Model file for the job. Use its own axes, mm. A direction names the side the tool comes from. Coordinates: 2 decimals unless noted, no trailing zeros. Loops run counter-clockwise (first coordinate to the right, second up) from the corner with the lowest first, then second, coordinate; pieces in that order, holes last. Notation, with made-up numbers: (76, 69.25) -> (87, 69.25) arc R10 cw to (87, 87.25) -> close; hole circle Ø5 at (5, -3.5). An arc over 180 degrees is marked (long way). Use one line per item in the form item = value.
```python
from build123d import *

# Parameters (mm, degrees)
MODEL_W             = 8.001
MODEL_H             = 8.001
BOSS_EXTRUDE2_DEPTH = 6.35


with BuildPart() as part:
    # Model → Boss-Extrude2 (new body)
    with BuildSketch(Plane.XY):
        Polygon((419.1, 87.376), (419.1, 71.374), (436.88, 71.374), (436.88, 63.5), (398.78, 0), (0, 0), (0, 95.25), (436.88, 95.25), (436.88, 87.376), align=None)
        with Locations((70.891200524, 88.9)):
            Rectangle(MODEL_W, MODEL_H, mode=Mode.SUBTRACT)
        Polygon((235.853706977, 81.865965064), (235.938184476, 73.865411048), (227.937630461, 73.780933549), (227.853152962, 81.781487564), align=None, mode=Mode.SUBTRACT)
        with BuildLine():
            Line((171.232102448, 6.35), (215.9, 6.35))
            ThreePointArc((215.9, 6.35), (220.390128061, 8.209871939), (222.25, 12.7))
            Line((222.25, 12.7), (222.25, 57.367897552))
            ThreePointArc((222.25, 57.367897552), (220.682015918, 59.714551565), (217.913948776, 59.163948776))
            Line((217.913948776, 59.163948776), (169.436051224, 10.686051224))
            ThreePointArc((169.436051224, 10.686051224), (168.885448435, 7.917984082), (171.232102448, 6.35))
        make_face(mode=Mode.SUBTRACT)
        with BuildLine():
            Line((234.95, 57.367897552), (234.95, 12.7))
            ThreePointArc((234.95, 12.7), (236.809871939, 8.209871939), (241.3, 6.35))
            Line((241.3, 6.35), (285.967897552, 6.35))
            ThreePointArc((285.967897552, 6.35), (288.314551565, 7.917984082), (287.763948776, 10.686051224))
            Line((287.763948776, 10.686051224), (239.286051224, 59.163948776))
            ThreePointArc((239.286051224, 59.163948776), (236.517984082, 59.714551565), (234.95, 57.367897552))
        make_face(mode=Mode.SUBTRACT)
        with BuildLine():
            Line((294.113948776, 17.036051224), (245.636051224, 65.513948776))
            ThreePointArc((245.636051224, 65.513948776), (245.085448435, 68.282015918), (247.432102448, 69.85))
            Line((247.432102448, 69.85), (292.1, 69.85))
            ThreePointArc((292.1, 69.85), (296.590128061, 67.990128061), (298.45, 63.5))
            Line((298.45, 63.5), (298.45, 18.832102448))
            ThreePointArc((298.45, 18.832102448), (296.882015918, 16.485448435), (294.113948776, 17.036051224))
        make_face(mode=Mode.SUBTRACT)
        with BuildLine():
            Line((323.632102448, 6.35), (368.3, 6.35))
            ThreePointArc((368.3, 6.35), (372.790128061, 8.209871939), (374.65, 12.7))
            Line((374.65, 12.7), (374.65, 57.367897552))
            ThreePointArc((374.65, 57.367897552), (373.082015918, 59.714551565), (370.313948776, 59.163948776))
            Line((370.313948776, 59.163948776), (321.836051224, 10.686051224))
            ThreePointArc((321.836051224, 10.686051224), (321.285448435, 7.917984082), (323.632102448, 6.35))
        make_face(mode=Mode.SUBTRACT)
        with BuildLine():
            Line((18.832102448, 6.35), (63.5, 6.35))
            ThreePointArc((63.5, 6.35), (67.990128061, 8.209871939), (69.85, 12.7))
            Line((69.85, 12.7), (69.85, 57.367897552))
            ThreePointArc((69.85, 57.367897552), (68.282015918, 59.714551565), (65.513948776, 59.163948776))
            Line((65.513948776, 59.163948776), (17.036051224, 10.686051224))
            ThreePointArc((17.036051224, 10.686051224), (16.485448435, 7.917984082), (18.832102448, 6.35))
        make_face(mode=Mode.SUBTRACT)
        with BuildLine():
            Line((82.55, 57.367897552), (82.55, 12.7))
            ThreePointArc((82.55, 12.7), (84.409871939, 8.209871939), (88.9, 6.35))
            Line((88.9, 6.35), (133.567897552, 6.35))
            ThreePointArc((133.567897552, 6.35), (135.914551565, 7.917984082), (135.363948776, 10.686051224))
            Line((135.363948776, 10.686051224), (86.886051224, 59.163948776))
            ThreePointArc((86.886051224, 59.163948776), (84.117984082, 59.714551565), (82.55, 57.367897552))
        make_face(mode=Mode.SUBTRACT)
        with BuildLine():
            Line((93.236051224, 65.513948776), (141.713948776, 17.036051224))
            ThreePointArc((141.713948776, 17.036051224), (144.482015918, 16.485448435), (146.05, 18.832102448))
            Line((146.05, 18.832102448), (146.05, 63.5))
            ThreePointArc((146.05, 63.5), (144.190128061, 67.990128061), (139.7, 69.85))
            Line((139.7, 69.85), (95.032102448, 69.85))
            ThreePointArc((95.032102448, 69.85), (92.685448435, 68.282015918), (93.236051224, 65.513948776))
        make_face(mode=Mode.SUBTRACT)
        with BuildLine():
            Line((163.086051224, 17.036051224), (211.563948776, 65.513948776))
            ThreePointArc((211.563948776, 65.513948776), (212.114551565, 68.282015918), (209.767897552, 69.85))
            Line((209.767897552, 69.85), (165.1, 69.85))
            ThreePointArc((165.1, 69.85), (160.609871939, 67.990128061), (158.75, 63.5))
            Line((158.75, 63.5), (158.75, 18.832102448))
            ThreePointArc((158.75, 18.832102448), (160.317984082, 16.485448435), (163.086051224, 17.036051224))
        make_face(mode=Mode.SUBTRACT)
        with BuildLine():
            Line((315.486051224, 17.036051224), (363.963948776, 65.513948776))
            ThreePointArc((363.963948776, 65.513948776), (364.514551565, 68.282015918), (362.167897552, 69.85))
            Line((362.167897552, 69.85), (317.5, 69.85))
            ThreePointArc((317.5, 69.85), (313.009871939, 67.990128061), (311.15, 63.5))
            Line((311.15, 63.5), (311.15, 18.832102448))
            ThreePointArc((311.15, 18.832102448), (312.717984082, 16.485448435), (315.486051224, 17.036051224))
        make_face(mode=Mode.SUBTRACT)
        with BuildLine():
            Line((6.35, 63.5), (6.35, 18.832102448))
            ThreePointArc((6.35, 18.832102448), (7.917984082, 16.485448435), (10.686051224, 17.036051224))
            Line((10.686051224, 17.036051224), (59.163948776, 65.513948776))
            ThreePointArc((59.163948776, 65.513948776), (59.714551565, 68.282015918), (57.367897552, 69.85))
            Line((57.367897552, 69.85), (12.7, 69.85))
            ThreePointArc((12.7, 69.85), (8.209871939, 67.990128061), (6.35, 63.5))
        make_face(mode=Mode.SUBTRACT)
    extrude(amount=BOSS_EXTRUDE2_DEPTH)


solid = part.part
```
Q1. Which spindle directions (+Z, -Z, +X, -X, +Y, -Y) get a long thin tool onto all of the face, cutting with end or side? Do faces 1 (the face through (346.41, 35.26, 3.13)), 2 (the face through (221, 69, 0)). Say none if no direction does.
Result:
face_1 = +Z, -Z
face_2 = -Z, +X, -X, +Y, -Y
Q2. Mould opens along X. For faces 3 (the face through (418.1, 32.2, 3.1)), 4 (the face through (221, 69, 6.35)), 5 (the face through (270.21, 40.94, 3.13)) say: released by +X, released by -X, zero draft, split by the parting line, or undercut.
Result:
face_3 = released by +X
face_4 = zero draft
face_5 = undercut
Q3. Band-saw the part on D-D, the plane x = 48. Write the cut outline in (y, z).
Result:
outline = (0, 0) -> (6.35, 0) -> (6.35, 6.35) -> (0, 6.35) -> close; (41.65, 0) -> (54.35, 0) -> (54.35, 6.35) -> (41.65, 6.35) -> close; (69.85, 0) -> (95.25, 0) -> (95.25, 6.35) -> (69.85, 6.35) -> close
Q4. Band-saw the part on B-B, the plane y = 27. State how many separate pieces and enclosed holes the cut face has, and give its area (3 significant figures).
Result:
separate_pieces = 11
enclosed_holes = 0
area = 1,020 mm2
Q5. Pin check, flat tips, straight feed: pin 1 Ø10 at (x, y) = (266.5, 32.5) entering from -Z; pin 2 Ø1.9 at (y, z) = (35, 4) entering from +X. Stop position of each tip, or through.
Result:
pin_1 = 0
pin_2 = 420.35
Q6. Band-saw the part on A-A, the plane x = 103.5. Write the cut outline in (y, z).
Result:
outline = (0, 0) -> (6.35, 0) -> (6.35, 6.35) -> (0, 6.35) -> close; (42.55, 0) -> (55.25, 0) -> (55.25, 6.35) -> (42.55, 6.35) -> close; (69.85, 0) -> (95.25, 0) -> (95.25, 6.35) -> (69.85, 6.35) -> close
Q7. Wall check: line 1 along Y through (x, z) = (326, 4.5); line 2 along X through (y, z) = (66, 1.5); line 3 along Y through (x, z) = (31, 4.75). Give the ranges that are in metal, low to high.
Result:
line_1 = 0 to 6.35, 14.85 to 27.55, 69.85 to 95.25
line_2 = 0 to 6.86, 59.54 to 92.86, 145.54 to 159.26, 211.94 to 245.26, 297.94 to 311.66, 364.34 to 436.88
line_3 = 0 to 6.35, 24.65 to 37.35, 69.85 to 95.25
